Build history of the part. All positions in model axes, mm. Face numbers are marked on the shaded views. A direction names the side the tool comes from. Coordinates: 2 decimals unless noted, no trailing zeros. Loops run counter-clockwise (first coordinate to the right, second up) from the corner with the lowest first, then second, coordinate; pieces in that order, holes last.
Item 1: Cut at B-B (x = 25.5). List the corners of the cut face in (y, z) (3 decimals).
Item 2: 3-axis set-ups, long thin cutter, end or side, ignore diameter. For the marked faces 4 and 5: which of +Z, -Z, +X, -X, +Y, -Y reach the whole face in a straight line?
Item 3: Cut at C-C (z = -16.5). List the corners of the cut face in (x, y) (3 decimals), and give its area (3 significant figures).
Item 4: Mould opens along Z. For the marked faces 1, 2 and 3 say: released by +Z, released by -Z, zero draft, split by the parting line, or undercut.
Item 5: Cut at D-D (x = 89). List the corners of the cut face in (y, z) (3 decimals), and give its area (3 significant figures).
Item 6: Drill centre lines: line 1 along Y through (x, z) = (39.5, -40) (3 decimals); line 2 along Z through (x, y) = (7, 22) (3 decimals). Where is each one in solid material? Low to high.
Item 7: Cut at A-A (y = 10.5). List the corners of the cut face in (x, z) (3 decimals), and give its area (3 significant figures).
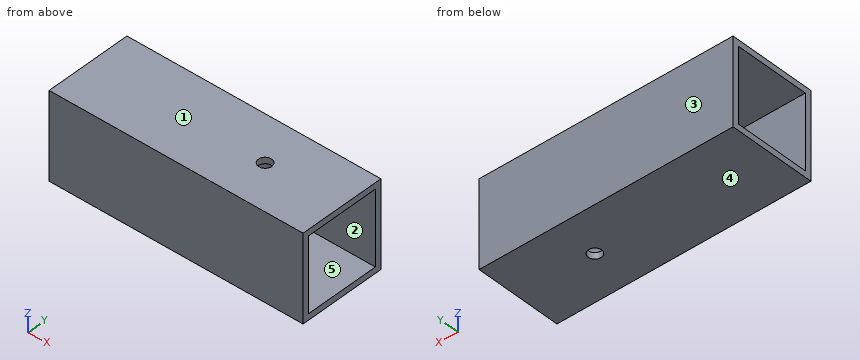
from build123d import *

# Parameters (mm, degrees)
SKETCH2_W               = 44.45
SKETCH2_H               = 44.45
SKETCH2_W_2             = 38.1
SKETCH2_H_2             = 38.1
BOSS_EXTRUDE1_DEPTH     = 130.048
F_1_4_CLEARANCE_HOLE1_D = 6.7564


with BuildPart() as part:
    # Sketch2 → Boss-Extrude1 (new body)
    with BuildSketch(Plane(origin=(0, 0, 0), x_dir=(0, 0, -1), z_dir=(1, 0, 0))):
        with Locations((22.225, 22.225)):
            Rectangle(SKETCH2_W, SKETCH2_H)
        with Locations((22.225, 22.225)):
            Rectangle(SKETCH2_W_2, SKETCH2_H_2, mode=Mode.SUBTRACT)
    extrude(amount=BOSS_EXTRUDE1_DEPTH)

    # 1/4 Clearance Hole1 (through all)
    with Locations(Plane.XY):
        with Locations((90.678, 22.225)):
            Hole(F_1_4_CLEARANCE_HOLE1_D / 2)


solid = part.part
Filled sheet:
1. outline: (0, -44.45) - (44.45, -44.45) - (44.45, 0) - (0, 0) - close; hole (3.175, -41.275) - (41.275, -41.275) - (41.275, -3.175) - (3.175, -3.175) - close
2. face 4: -Z, +X, -X, +Y, -Y
2. face 5: +X, -X
3. outline: (0, 0) - (130.048, 0) - (130.048, 3.175) - (0, 3.175) - close; (0, 41.275) - (130.048, 41.275) - (130.048, 44.45) - (0, 44.45) - close
3. area: 826 mm2
4. face 1: released by +Z
4. face 2: undercut
4. face 3: zero draft
5. outline: (0, -44.45) - (19.293, -44.45) - (19.293, -41.275) - (3.175, -41.275) - (3.175, -3.175) - (19.293, -3.175) - (19.293, 0) - (0, 0) - close; (25.157, -44.45) - (44.45, -44.45) - (44.45, 0) - (25.157, 0) - (25.157, -3.175) - (41.275, -3.175) - (41.275, -41.275) - (25.157, -41.275) - close
5. area: 487 mm2
6. line 1: y = 0 to 3.175, 41.275 to 44.45
6. line 2: z = -44.45 to -41.275, -3.175 to 0
7. outline: (0, -44.45) - (130.048, -44.45) - (130.048, -41.275) - (0, -41.275) - close; (0, -3.175) - (130.048, -3.175) - (130.048, 0) - (0, 0) - close
7. area: 826 mm2
